Autodesk Inventor part; units mm, degrees
ref_plane "YZ Plane" through (0, 0, 0) normal (1, 0, 0) x (0, 1, 0)
ref_plane "XZ Plane" through (0, 0, 0) normal (0, 1, 0) x (-1, 0, 0)
ref_plane "XY Plane" through (0, 0, 0) normal (0, 0, 1) x (1, 0, 0)
sketch "Sketch1" plane through (0, 0, 0) normal (0, 0, 1) x (1, 0, 0)
  line L0 (0, 0) -> (247.65, 0)
  line L1 (247.65, 0) -> (247.65, 38.1)
  line L2 (247.65, 38.1) -> (0, 38.1)
  line L3 (0, 38.1) -> (0, 0)
  line L4 (286.1616, 0) -> (255.1962, 0)
  line L5 (255.1962, 0) -> (255.1962, 12.7)
  line L6 (255.1962, 12.7) -> (286.1616, 12.7)
  line L7 (286.1616, 12.7) -> (286.1616, 0)
  line L8 (247.65, 12.7) -> (200.66, 12.7)
  circle A0 centre (200.6294, 0) radius 47.0206
  line L9 (16.2468, 38.1) -> (16.2468, 12.7)
  line L10 (16.2468, 12.7) -> (155.3565, 12.7)
  line L11 (0, 12.7) -> (17.7951, 12.7)
  line L12 (179.5891, -42.0504) -> (75.8552, 12.7)
  dimension "d0" = 247.65
  dimension "d1" = 38.1
  dimension "d2" = 12.7
  dimension "d3" = 30.9654
  dimension "d4" = 46.99
extrude "Extrusion1" add sketch "Sketch1" along normal blind 1.5875 contours L12 L10 A0 L0 | L0 A0 L12 | L3 L2 L9 L11 | A0 L2 L0 | L0 A0 L12 | L10 L9 L2 A0 | A0 L8 L1 | L8 A0 L2 L1
fillet "Fillet1" radius 28.575 1 edges at (247.65, 38.1, 0.7937)
fillet "Fillet2" radius 3.175 1 edges at (0, 38.1, 0.7937)
fillet "Fillet3" radius 3.175 1 edges at (0, 12.7, 0.7937)
properties part number "intake sled v5"
Geometry: final body of the model. Coordinates: model frame, mm. Coordinates: 2 decimals unless noted, no trailing zeros. Order: outer loops, then holes, each group sorted by start corner. A loop starts at its lowest first (then second) coordinate and runs counter-clockwise, first axis right, second up. Notation, with made-up numbers: (79, -30.5) - (112, -30.5) arc R13 cw to (112, -14.5) - close; hole circle Ø9 at (38.5, -1.5). An arc over 180 degrees is marked (long way). Write each question's results on one line, items separated by ' | '.
(1) Section query A-A, the plane z = 0.25. Return the cut outline in (x, y) (3 decimals).
Values found:
outline: (0, 15.875) arc R3.175 ccw to (3.175, 12.7) - (75.855, 12.7) - (179.589, -42.05) arc R47.021 ccw to (247.65, 0) - (247.65, 9.525) arc R28.575 ccw to (219.075, 38.1) - (3.175, 38.1) arc R3.175 ccw to (0, 34.925) - close
(2) Section query C-C, the plane y = -18. Return the cut outline in (x, z), plus the area to 3 significant figures.
Values found:
outline: (134.02, 0) - (244.07, 0) - (244.07, 1.59) - (134.02, 1.59) - close | area: 175 mm²
(3) Line query: line 1 (Y direction, x = 44.5, z = 1.1); line 2 (X direction, y = -7, z = 1.1); line 3 (X direction, y = 22.5, z = 0.7). Output: solid intervals per line, ascending. Write a range as [from, to].
Values found:
line 1: y = [12.7, 38.1] | line 2: x = [113.18, 247.13] | line 3: x = [0, 244.53]
(4) Section query B-B, the plane x = 46.5. Return the cut outline in (y, z).
Values found:
outline: (12.7, 0) - (38.1, 0) - (38.1, 1.59) - (12.7, 1.59) - close
